The listing builds one solid part. Answer for the finished solid, in the listing's coordinates (mm). A direction names the side the tool comes from. Give positions to 0.01 mm unless a question says otherwise; leave off trailing zeros. Loops run counter-clockwise (first coordinate to the right, second up) from the corner with the lowest first, then second, coordinate; pieces in that order, holes last. Notation, with made-up numbers: (42.25, -21) - (98.25, -21) arc R22 ccw to (98.25, 15) - close; hole circle Ø2 at (19, 50.25). An arc over 180 degrees is marked (long way). Answer in a Markdown table with one row per item. Add a question column.
Autodesk Inventor part; units mm, degrees
ref_plane "YZ Plane" through (0, 0, 0) normal (1, 0, 0) x (0, 1, 0)
ref_plane "XZ Plane" through (0, 0, 0) normal (0, 1, 0) x (-1, 0, 0)
ref_plane "XY Plane" through (0, 0, 0) normal (0, 0, 1) x (1, 0, 0)
sketch "Sketch1" plane through (0, 0, 0) normal (0, 0, 1) x (1, 0, 0)
  circle A0 centre (0, 0) radius 26.797
  line L0 (-26.797, -45.7454) -> (26.797, -45.7454)
  line L1 (-26.797, 0) -> (-26.797, -45.7454)
  line L2 (26.797, 0) -> (26.797, -45.7454)
  line L3 (-26.797, -45.7454) -> (26.797, -45.7454)
  point P0 (0, 0)
extrude "Extrusion1" add sketch "Sketch1" along normal blind 1.5875
sketch "Sketch2" plane through (0, 0, 1.5875) normal (0, 0, 1) x (1, 0, 0)
  line L0 (26.797, 0) -> (26.797, -45.7454)
  line L1 (-26.797, -45.7454) -> (26.797, -45.7454)
  line L2 (26.797, -45.7454) -> (26.797, -44.1579)
  line L3 (26.797, -44.1579) -> (-26.797, -44.1579)
  line L4 (-26.797, -44.1579) -> (-26.797, -45.7454)
  dimension "d2" = 1.5875
extrude "Extrusion2" add sketch "Sketch2" along normal blind 12.7
fillet "Fillet1" radius 3.175 2 edges at (-26.797, -44.9517, 14.2875) (26.797, -44.9517, 14.2875)
hole "Hole1" at (-20.447, -44.1579, 7.9375) direction (0, -1, 0) diameter 5.1054 end through all
fillet "Fillet2" radius 0.7937 1 edges at (0, -44.1579, 1.5875)
hole "Hole2" at (20.447, -44.1579, 7.9375) direction (0, -1, 0) diameter 5.1054 end through all
sketch "Sketch3" plane through (0, 0, 1.5875) normal (0, 0, 1) x (1, 0, 0)
  arc A0 (26.797, 0) -> (-26.797, 0) centre (0, 0) ccw
  point P0 (-19.05, 0)
  point P1 (19.05, 0)
  dimension "d26" = 19.05
  dimension "d27" = 19.05
hole "Hole3" at (-19.05, 0, 1.5875) at (19.05, 0, 1.5875) direction (0, 0, -1) diameter 3.81 end through all
fillet "Fillet3" radius 3.175 1 edges at (0, -45.7454, 0)
properties part number "Pneumatics_VIAIR_00090_02"
(1) Given pin 1 Ø8 at (y, z) = (4.5, 5) entering from -X; pin 2 Ø6 at (x, z) = (-5, 9.5) entering from +Y; pin 3 Ø4.5 at (x, y) = (-19.05, 0) entering from +Z, each flat-ended and moving along its own axis, determine where each tip first touches the part or whether it passes through.
(2) A cutting plane is placed at C-C on z = 13.25. Determine the outline of the cut face in (x, y), plus the area to 3 significant figures.
(3) The mould has two halves that part along Z. Classify faces 1 (the face through (22, -44.96, 5.91)), 2 (the face through (0.375, -44.84, 0.955)), 3 (the face through (0, -45.745, 9)): pulls with the +Z half, pulls with the -Z half, needs draft (parallel to the pull), parting line crosses it, or undercut.
(4) Find the intervals of material crossed by line 1 along X through (y, z) = (0, 0.65) (3 decimals); line 2 along Z through (x, y) = (13, -12.5); line 3 along Y through (x, z) = (21, 10.75), in increasing order. Write a range as [from, to].
(5) A cutting plane is placed at D-D on y = -19. Determine the outline of the cut face in (x, z), plus the area to 3 significant figures.
(6) A cutting plane is placed at B-B on x = -19.05. Give the number of separate pieces and of enclosed holes in the cut face, plus the area to 3 significant figures.
(7) A tool of negligible diameter and unlimited length cuts with its end or side. For faces 4 (the face through (0, -8, 1.588)), 5 (the face through (26.797, -26, 1)), from which of +Z, -Z, +X, -X, +Y, -Y can it reach the whole face along a straight path? Write none if from no direction.
Evaluation:
| question | item | result |
|---|---|---|
| 1 | pin 1 | stops at x = -26.69 |
| 1 | pin 2 | stops at y = -44.16 |
| 1 | pin 3 | stops at z = 1.59 |
| 2 | outline | (-25.97, -45.75) - (25.97, -45.75) - (25.97, -44.16) - (-25.97, -44.16) - close |
| 2 | area | 82.5 mm² |
| 3 | face 1 | undercut |
| 3 | face 2 | pulls with the -Z half |
| 3 | face 3 | needs draft |
| 4 | line 1 | x = [-26.797, -20.955], [-17.145, 17.145], [20.955, 26.797] |
| 4 | line 2 | z = [0, 1.59] |
| 4 | line 3 | y = [-45.75, -44.16] |
| 5 | outline | (-26.8, 0) - (26.8, 0) - (26.8, 1.59) - (-26.8, 1.59) - close |
| 5 | area | 85.1 mm² |
| 6 | separate pieces | 3 |
| 6 | enclosed holes | 0 |
| 6 | area | 108 mm² |
| 7 | face 4 | +Z, +X, -X, +Y |
| 7 | face 5 | +Z, -Z, +X, +Y, -Y |
